Can you work these out from the drawing? Everything is in mm from the part's minimum corner. Round coordinates to 2 decimals unless told otherwise and drop trailing zeros. Write each loop counter-clockwise with the first axis right and the second up, starting at its lowest first coordinate (ties: lowest second). Pieces come first, ordered by that corner, then holes. Notation, with made-up numbers: (26.25, 37.25) -> (30.25, 37.25) arc R29 ccw to (30.25, 63.25) -> close; hole circle Ø7 at (62, -37.75). An arc over 180 degrees is marked (long way). Answer as CSV lines item,"result".
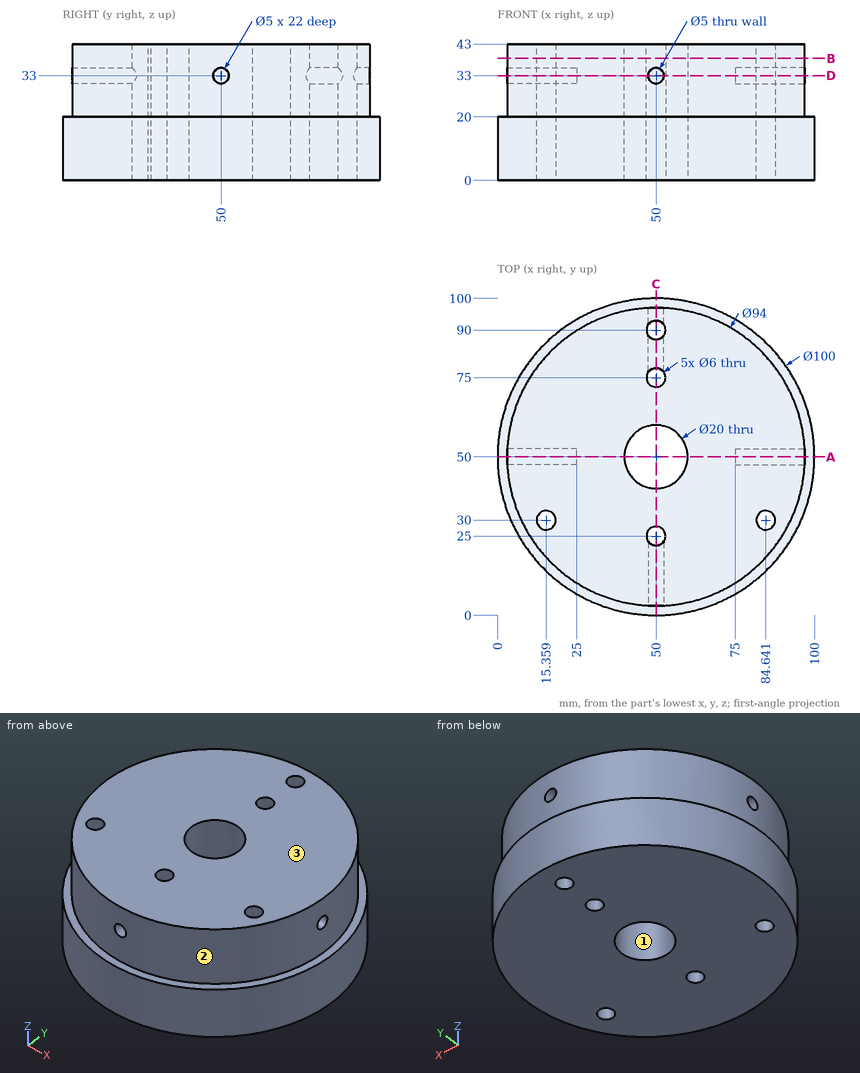
Item 1: Suppose I cut it at D-D, the plane z = 33. List the corners of the cut face in (x, y) for me, then the cut area to 3 significant figures.
Results found:
outline,"(3.07, 47.5) arc R47 ccw to (47.5, 3.07) -> (47.5, 23.34) arc R3 cw (long way) to (52.5, 23.34) -> (52.5, 3.07) arc R47 ccw to (96.93, 47.5) -> (75, 47.5) -> (75, 52.5) -> (96.93, 52.5) arc R47 ccw to (52.5, 96.93) -> (52.5, 91.66) arc R3 cw to (52.5, 88.34) -> (52.5, 76.66) arc R3 cw (long way) to (47.5, 76.66) -> (47.5, 88.34) arc R3 cw to (47.5, 91.66) -> (47.5, 96.93) arc R47 ccw to (3.07, 52.5) -> (25, 52.5) -> (25, 47.5) -> close; hole circle Ø6 at (15.36, 30); hole circle Ø20 at (50, 50); hole circle Ø6 at (84.64, 30)"
area,"6,100 mm²"
Item 2: I need wall thicknesses on L1, parallel to Y at x = 82, z = 33; L2, parallel to Z at x = 50, y = 94; L3, parallel to Y at x = 52.5, z = 16. Which ranges of each line are inside material? Lowest first, please.
Results found:
L1,"y = 15.58 to 28.58, 31.42 to 47.5, 52.5 to 84.42"
L2,"z = 0 to 30.5, 35.5 to 43"
L3,"y = 0.06 to 23.34, 26.66 to 40.32, 59.68 to 73.34, 76.66 to 88.34, 91.66 to 99.94"
Item 3: Suppose I cut it at B-B, the plane z = 38.5. List the corners of the cut face in (x, y) for me.
Results found:
outline,"circle Ø94 at (50, 50); hole circle Ø6 at (15.36, 30); hole circle Ø20 at (50, 50); hole circle Ø6 at (50, 25); hole circle Ø6 at (50, 75); hole circle Ø6 at (50, 90); hole circle Ø6 at (84.64, 30)"
Item 4: Suppose I cut it at A-A, the plane y = 50. List the corners of the cut face in (x, z) for me.
Results found:
outline,"(0, 0) -> (40, 0) -> (40, 43) -> (3, 43) -> (3, 35.5) -> (25, 35.5) -> (25, 30.5) -> (3, 30.5) -> (3, 20) -> (0, 20) -> close; (60, 0) -> (100, 0) -> (100, 20) -> (97, 20) -> (97, 30.5) -> (75, 30.5) -> (75, 35.5) -> (97, 35.5) -> (97, 43) -> (60, 43) -> close"
Item 5: If we mould it in two halves opening along X, with no side actions, what happens to the marked faces 1, 2 and 3? For each: pulls with the +X half, pulls with the -X half, needs draft (parallel to the pull), parting line crosses it, or undercut.
Results found:
face 1,"undercut"
face 2,"parting line crosses it"
face 3,"needs draft"
Item 6: Suppose I cut it at C-C, the plane x = 50. State how many separate pieces and enclosed holes the cut face has, then the cut area to 3 significant figures.
Results found:
separate pieces,"8"
enclosed holes,"0"
area,"2,370 mm²"
Item 7: Will these pins go through, and if not, where does the flat tip stop? pin 1 (10 mm diameter, centred on y = 85.5, z = 11, fed in from +X); pin 2 (3 mm diameter, centred on x = 50, z = 33, fed in from +Y); pin 3 (6 mm diameter, centred on x = 50, z = 33, fed in from +Y).
Results found:
pin 1,"stops at x = 89.62"
pin 2,"stops at y = 72.4"
pin 3,"stops at y = 97"
